from build123d import *

# Parameters (mm, degrees)
SKETCH_1_W               = 76
SKETCH_1_H               = 67
SKETCH_1_R               = 3.5
EXTRUDE_1_DEPTH          = 8
SKETCH_2_W               = 44
SKETCH_2_H               = 44
SKETCH_2_W_2             = 40
SKETCH_2_H_2             = 40
EXTRUDE_1_2_DEPTH        = 50
CUT_EXTRUDE_1_REACH      = 90.816
SKETCH_3_R               = 2.75
PATTERN_CIRCULAR_1_COUNT = 4


with BuildPart() as part:
    # Sketch 1 → Extrude 1 (new body)
    with BuildSketch(Plane(origin=(0, 0, 0), x_dir=(1, 0, 0), z_dir=(0, 1, 0))):
        Rectangle(SKETCH_1_W, SKETCH_1_H)
        with Locations(Location((-25, 21, 0), (0, 0, 270))):
            Circle(SKETCH_1_R, mode=Mode.SUBTRACT)
        with Locations(Location((25, 21, 0), (0, 0, 90))):
            Circle(SKETCH_1_R, mode=Mode.SUBTRACT)
        with Locations(Location((25, -21, 0), (0, 0, 270))):
            Circle(SKETCH_1_R, mode=Mode.SUBTRACT)
        with Locations(Location((-25, -21, 0), (0, 0, 90))):
            Circle(SKETCH_1_R, mode=Mode.SUBTRACT)
    extrude(amount=EXTRUDE_1_DEPTH)

    # Sketch 2 → Extrude 1 2 (add)
    with BuildSketch(Plane(origin=(0, 8, 0), x_dir=(1, 0, 0), z_dir=(0, 1, 0))):
        Rectangle(SKETCH_2_W, SKETCH_2_H)
        Rectangle(SKETCH_2_W_2, SKETCH_2_H_2, mode=Mode.SUBTRACT)
    extrude(amount=EXTRUDE_1_2_DEPTH)

    # Sketch 3 → Cut-Extrude 1 (cut, up to next)
    with BuildSketch(Plane.XY.offset(22), mode=Mode.PRIVATE) as cut_extrude_1_sk1:
        with Locations((0, 38)):
            Circle(SKETCH_3_R)
    cut_extrude_1_tool1 = extrude(cut_extrude_1_sk1.sketch, amount=-CUT_EXTRUDE_1_REACH, mode=Mode.PRIVATE) & part.part
    cut_extrude_1 = cut_extrude_1_tool1.solids().sort_by_distance((0, 38, 22))[0]
    add(cut_extrude_1, mode=Mode.SUBTRACT)

    # Pattern Circular 1: Cut-Extrude 1 ×4 about axis
    pattern_circular_1_axis = Axis((0, 55, 0), (0, -1, 0))
    for i in range(1, PATTERN_CIRCULAR_1_COUNT):
        add(cut_extrude_1.rotate(pattern_circular_1_axis, i * 360 / PATTERN_CIRCULAR_1_COUNT), mode=Mode.SUBTRACT)


solid = part.part
Can you work these out from the model? Positions are in its coordinate system, mm. A direction names the side the tool comes from. Give positions to 0.01 mm unless a question says otherwise; leave off trailing zeros. Order: outer loops, then holes, each group sorted by start corner. A loop starts at its lowest first (then second) coordinate and runs counter-clockwise, first axis right, second up. Notation, with made-up numbers: M 58,21 L 100,21 A26 cw 100,49 Z; hole C -9.75,-25.75 d3. An arc over 180 degrees is marked long. Use one line per item in the form item = value. Start each with the question number.
Item 1: Will these pins go through, and if not, where does the flat tip stop? pin 1 Ø6.5 at (y, z) = (38, 0) entering from +X; pin 2 Ø6 at (y, z) = (25.5, -20) entering from -X; pin 3 Ø2 at (x, y) = (-3.5, 29.5) entering from -Z.
Item 2: If we section it at A-A (z = 21): Write out the boundary of the cut face in (x, y), then the cut area to 3 significant figures.
Item 3: If we section it at B-B (x = -25): Write out the boundary of the cut face in (y, z), then the cut area to 3 significant figures.
Item 4: If we section it at D-D (z = 0): Write out the boundary of the cut face in (x, y), then the cut area to 3 significant figures.
Item 5: We'd pull the mould along Y, two halves only. Please class faces 1 (the flat face through (-1, 0, 0)), 2 (the cylindrical face through (-22.05, 3.94, -19.12)), 3 (the cylindrical face through (-0.358, 40.727, 21.014)): +Y half, -Y half, draft (parallel to the pull), parting line (faces both ways), or undercut.
Item 6: For faces 4 (the flat face through (22, 33, 0)), 5 (the flat face through (0, 33, -22)), 6 (the flat face through (-22, 33, 0)), which set-ups out of +Z, -Z, +X, -X, +Y, -Y let a thin tool reach every point of the face, with its end or its side?
Item 7: If I drill on line 1 along X through (y, z) = (3, -21); line 2 along Z through (x, y) = (15, 35); line 3 along Y through (x, z) = (-20.7, 0), over which ranges is the centre line in solid material (lowest first)?
Item 8: If we section it at C-C (y = 34): Write out the boundary of the cut face in (x, z).
Outcome:
q1.pin_1 = 22
q1.pin_2 = -22
q1.pin_3 = -22
q2.outline = M -38,0 L -28.5,0 L -28.5,8 L -38,8 Z; M -22,8 L -21.5,8 L -21.5,0 L 21.5,0 L 21.5,8 L 22,8 L 22,58 L -22,58 Z; M 28.5,0 L 38,0 L 38,8 L 28.5,8 Z; hole C 0,38 d5.5
q2.area = 2,670 mm2
q3.outline = M 0,-33.5 L 8,-33.5 L 8,-24.5 L 0,-24.5 Z; M 0,-17.5 L 8,-17.5 L 8,17.5 L 0,17.5 Z; M 0,24.5 L 8,24.5 L 8,33.5 L 0,33.5 Z
q3.area = 424 mm2
q4.outline = M -38,0 L 38,0 L 38,8 L 22,8 L 22,35.25 L 20,35.25 L 20,8 L -20,8 L -20,35.25 L -22,35.25 L -22,8 L -38,8 Z; M -22,40.75 L -20,40.75 L -20,58 L -22,58 Z; M 20,40.75 L 22,40.75 L 22,58 L 20,58 Z
q4.area = 786 mm2
q5.face_1 = -Y half
q5.face_2 = draft
q5.face_3 = undercut
q6.face_4 = +Z, -Z, +X, +Y
q6.face_5 = -Z, +X, -X, +Y
q6.face_6 = +Z, -Z, -X, +Y
q7.line_1 = -38 to -28.5, -21.5 to 21.5, 28.5 to 38
q7.line_2 = -22 to -20, 20 to 22
q7.line_3 = 0 to 35.25, 40.75 to 58
q8.outline = M -22,-22 L 22,-22 L 22,22 L -22,22 Z; hole M -20,-20 L 20,-20 L 20,20 L -20,20 Z
